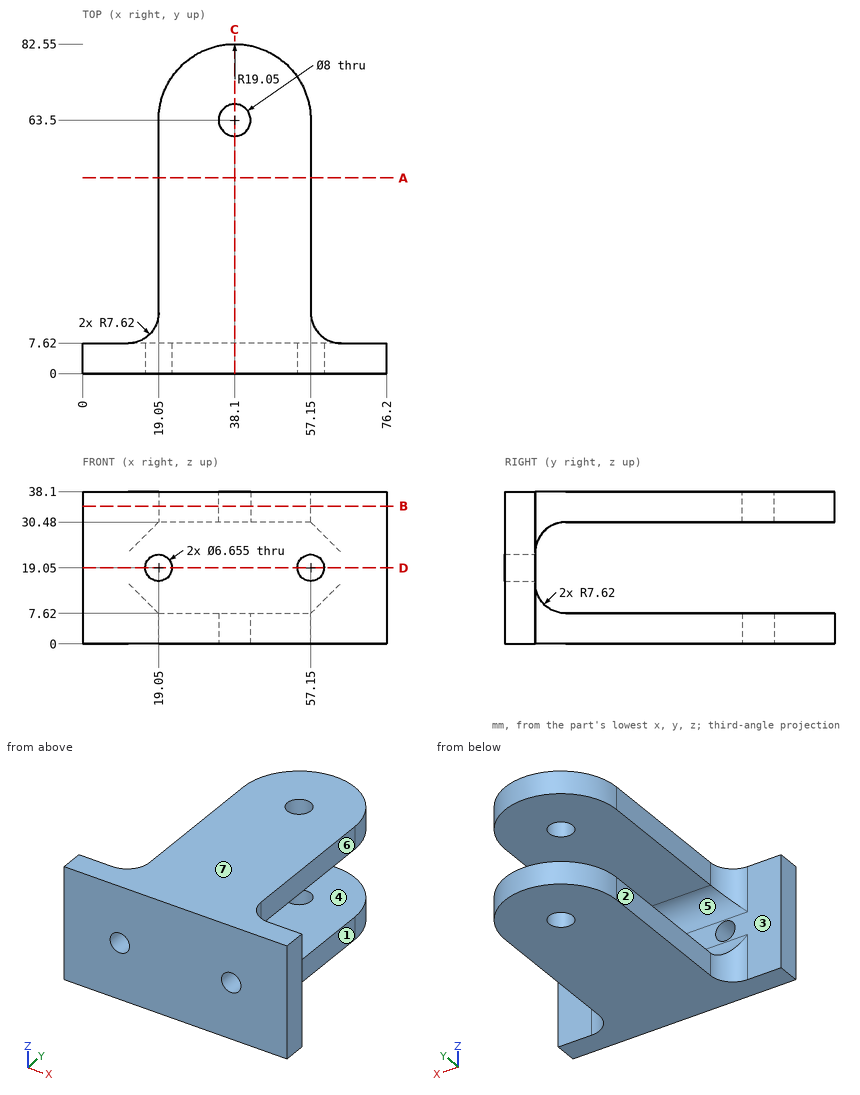
Source: three-view drawing plus pictorial views. Frame: mm from the lowest corner of the part. A direction names the side the tool comes from. Round coordinates to 2 decimals unless told otherwise and drop trailing zeros. Write each loop counter-clockwise with the first axis right and the second up, starting at its lowest first coordinate (ties: lowest second). Pieces come first, ordered by that corner, then holes. Notation, with made-up numbers: M -39,22 L 6,22 A17 cw 6,39 Z; hole C 41,71.5 d5. An arc over 180 degrees is marked long. Write item = value, one per line.
Item 1: Section query D-D on z = 19.05. Return loops of the section in (x, y).
Findings:
outline = M 0,0 L 15.72,0 L 15.72,7.62 L 0,7.62 Z; M 22.38,0 L 53.82,0 L 53.82,7.62 L 22.38,7.62 Z; M 60.48,0 L 76.2,0 L 76.2,7.62 L 60.48,7.62 Z
Item 2: Section query A-A on y = 49. Return loops of the section in (x, z).
Findings:
outline = M 19.05,0 L 57.15,0 L 57.15,7.62 L 19.05,7.62 Z; M 19.05,30.48 L 57.15,30.48 L 57.15,38.1 L 19.05,38.1 Z
Item 3: Material intervals for line 1 along X through (y, z) = (5.75, 19.05); line 2 along Z through (x, y) = (43, 25); line 3 along Z through (x, y) = (57, 4), sorted ascending. Write a range as [from, to].
Findings:
line_1 = [0, 15.72], [22.38, 53.82], [60.48, 76.2]
line_2 = [0, 7.62], [30.48, 38.1]
line_3 = [0, 15.73], [22.37, 38.1]
Item 4: Pin query (flat end, axial travel): P1, Ø6, axis at y = 27.5, z = 4.5, coming from the +X side; P2, Ø19, axis at x = 36.5, z = 24, coming from the +Y side; P3, Ø6, axis at y = 45, z = 2, coming from the -X side. Return the tip coordinate at first contact, or that it passes through.
Findings:
P1 = 57.15
P2 = 82.55
P3 = 19.05
Item 5: Section query C-C on x = 38.1. Return loops of the section in (y, z), then the cut area to 3 significant figures.
Findings:
outline = M 0,0 L 59.5,0 L 59.5,7.62 L 15.24,7.62 A7.62 cw 7.62,15.24 L 7.62,22.86 A7.62 cw 15.24,30.48 L 59.5,30.48 L 59.5,38.1 L 0,38.1 Z; M 67.5,0 L 82.55,0 L 82.55,7.62 L 67.5,7.62 Z; M 67.5,30.48 L 82.55,30.48 L 82.55,38.1 L 67.5,38.1 Z
area = 1,340 mm^2
Item 6: Section query B-B on z = 34.5. Return loops of the section in (x, y), then the cut area to 3 significant figures.
Findings:
outline = M 0,0 L 76.2,0 L 76.2,7.62 L 64.77,7.62 A7.62 cw 57.15,15.24 L 57.15,63.5 A19.05 ccw 19.05,63.5 L 19.05,15.24 A7.62 cw 11.43,7.62 L 0,7.62 Z; hole C 38.1,63.5 d8
area = 3,250 mm^2
Item 7: Access query for the marked faces 1, 2, 3 and 4. Directions: +Z, -Z, +X, -X, +Y, -Y. A direction counts if a zero-diameter tool reaches every point of the face in a straight line with its end or side. Return the directions, or none.
Findings:
face_1 = +Z, -Z, +X, +Y
face_2 = +Z, -Z, -X, +Y
face_3 = +Y
face_4 = +X, -X, +Y
Item 8: Pull-direction query (Z, two-part tool) for the marked faces 5, 6 and 7; classes: pulls with the +Z half, pulls with the -Z half, needs draft (parallel to the pull), parting line crosses it, or undercut.
Findings:
face_5 = undercut
face_6 = needs draft
face_7 = pulls with the +Z half
